```python
from build123d import *

# Parameters (mm, degrees)
SKETCH_1_R          = 11
EXTRUDE_1_DEPTH     = 2
EXTRUDE_START       = -2
SKETCH_3_R          = 1.55
EXTRUDE_2_DEPTH     = 2
CUT_EXTRUDE_1_REACH = 22.767
SKETCH_4_R          = 1.6
SKETCH_5_R          = 8.75
SKETCH_5_R_2        = 7.3
EXTRUDE_3_DEPTH     = 3


with BuildPart() as part:
    # 草图1 → 凸台-拉伸1 (new body)
    with BuildSketch(Plane(origin=(0, 0, 0), x_dir=(1, 0, 0), z_dir=(0, 1, 0))):
        with Locations(Location((0, 0, 0), (0, 0, 270))):
            Circle(SKETCH_1_R)
    extrude(amount=EXTRUDE_1_DEPTH)

    # 草图3 → 凸台-拉伸2 (add)
    # profile 1 of 2: a face of its own
    with BuildSketch(Plane(origin=(0, 2, 0), x_dir=(1, 0, 0), z_dir=(0, 1, 0)).offset(EXTRUDE_START)):
        with BuildLine():
            ThreePointArc((13.1875, 3.404385958), (11.2296215, 3.600530244), (9.814413265, 4.967624408))
            ThreePointArc((9.814413265, 4.967624408), (11, 0), (9.814413265, -4.967624408))
            ThreePointArc((9.814413265, -4.967624408), (11.2296215, -3.600530244), (13.1875, -3.404385958))
            ThreePointArc((13.1875, -3.404385958), (17.5, 0), (13.1875, 3.404385958))
        make_face()
        with Locations(Location((14, 0, 0), (0, 0, 270))):
            Circle(SKETCH_3_R, mode=Mode.SUBTRACT)
    # profile 2 of 2: a face of its own
    with BuildSketch(Plane(origin=(0, 2, 0), x_dir=(1, 0, 0), z_dir=(0, 1, 0)).offset(EXTRUDE_START)):
        with BuildLine():
            ThreePointArc((-9.814413265, 4.967624408), (-11, 0), (-9.814413265, -4.967624408))
            ThreePointArc((-9.814413265, -4.967624408), (-11.2296215, -3.600530244), (-13.1875, -3.404385958))
            ThreePointArc((-13.1875, -3.404385958), (-17.5, 0), (-13.1875, 3.404385958))
            ThreePointArc((-13.1875, 3.404385958), (-11.2296215, 3.600530244), (-9.814413265, 4.967624408))
        make_face()
        with Locations(Location((-14, 0, 0), (0, 0, 270))):
            Circle(SKETCH_3_R, mode=Mode.SUBTRACT)
    extrude(amount=EXTRUDE_2_DEPTH)

    # 草图4 → 切除-拉伸1 (cut, up to next)
    with BuildSketch(Plane.XZ, mode=Mode.PRIVATE) as cut_extrude_1_sk1:
        with Locations(Location((0, 0, 0), (0, 0, 270))):
            Circle(SKETCH_4_R)
    cut_extrude_1_tool1 = extrude(cut_extrude_1_sk1.sketch, amount=-CUT_EXTRUDE_1_REACH, mode=Mode.PRIVATE) & part.part
    add(cut_extrude_1_tool1.solids().sort_by_distance((0, 0, 0))[0], mode=Mode.SUBTRACT)

    # 草图5 → 凸台-拉伸3 (add)
    with BuildSketch(Plane(origin=(0, 2, 0), x_dir=(1, 0, 0), z_dir=(0, 1, 0))):
        with Locations(Location((0, 0, 0), (0, 0, 270))):
            Circle(SKETCH_5_R)
        with Locations(Location((0, 0, 0), (0, 0, 270))):
            Circle(SKETCH_5_R_2, mode=Mode.SUBTRACT)
    extrude(amount=EXTRUDE_3_DEPTH)


solid = part.part
```
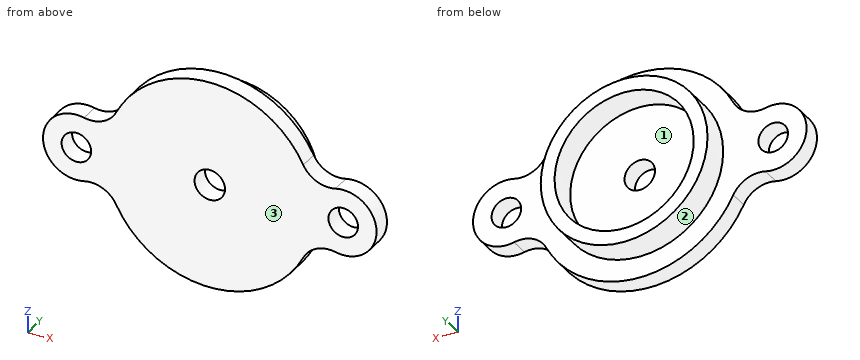
Geometry check sheet. Reference: the model listing, model coordinates, mm. Face numbers are marked on the shaded views. Give positions to 0.01 mm unless a question says otherwise; leave off trailing zeros. Order: outer loops, then holes, each group sorted by start corner. A loop starts at its lowest first (then second) coordinate and runs counter-clockwise, first axis right, second up.
1. Thickness scan on L1, parallel to X at y = 0.5, z = 0; L2, parallel to X at y = 1.45, z = -1.25; L3, parallel to X at y = 2.85, z = 0. Record the ranges inside material, lowest first.
2. Section check D-D, the plane x = 0. Enter the section's corners in (y, z), and give its area (3 significant figures).
3. Section check B-B, the plane y = 0.45. Enter the section's corners in (x, z), and give its area (3 significant figures).
4. Section check A-A, the plane x = -14. Enter the section's corners in (y, z).
5. Section check C-C, the plane z = -8. Enter the section's corners in (x, y).
6. Release check for a two-part mould opening along X. For the marked faces 1, 2 and 3 record: pulls with the +X half, pulls with the -X half, needs draft (parallel to the pull), parting line crosses it, or undercut.
7. Gauge pin test, flat ends, axial feed: pin 1 Ø1.5 at (y, z) = (3.5, -5) entering from +X; pin 2 Ø3.5 at (x, z) = (0, 0) entering from +Y. Record the tip position at first contact, or that the pin passes through.
Values follow:
1. L1: x = -17.5 to -15.55, -12.45 to -1.6, 1.6 to 12.45, 15.55 to 17.5
1. L2: x = -17.27 to -14.92, -13.08 to -1, 1 to 13.08, 14.92 to 17.27
1. L3: x = -8.75 to -7.3, 7.3 to 8.75
2. outline: (0, -11) - (2, -11) - (2, -8.75) - (5, -8.75) - (5, -7.3) - (2, -7.3) - (2, -1.6) - (0, -1.6) - close; (0, 1.6) - (2, 1.6) - (2, 7.3) - (5, 7.3) - (5, 8.75) - (2, 8.75) - (2, 11) - (0, 11) - close
2. area: 46.3 mm2
3. outline: (-13.19, -3.4) arc R3 cw to (-9.81, -4.97) arc R11 ccw to (9.81, -4.97) arc R3 cw to (13.19, -3.4) arc R3.5 ccw (long way) to (13.19, 3.4) arc R3 cw to (9.81, 4.97) arc R11 ccw to (-9.81, 4.97) arc R3 cw to (-13.19, 3.4) arc R3.5 ccw (long way) to start; hole circle Ø3.1 at (-14, 0); hole circle Ø3.2 at (0, 0); hole circle Ø3.1 at (14, 0)
3. area: 441 mm2
4. outline: (0, -3.5) - (2, -3.5) - (2, -1.55) - (0, -1.55) - close; (0, 1.55) - (2, 1.55) - (2, 3.5) - (0, 3.5) - close
5. outline: (-7.55, 0) - (7.55, 0) - (7.55, 2) - (3.54, 2) - (3.54, 5) - (-3.54, 5) - (-3.54, 2) - (-7.55, 2) - close
6. face 1: undercut
6. face 2: parting line crosses it
6. face 3: needs draft
7. pin 1: stops at x = 7.65
7. pin 2: stops at y = 2
